Work out the finished part from the listing and answer in its coordinate system (mm). A direction names the side the tool comes from. Round coordinates to 2 decimals unless told otherwise and drop trailing zeros. Loops run counter-clockwise (first coordinate to the right, second up) from the corner with the lowest first, then second, coordinate; pieces in that order, holes last.
```python
from build123d import *

# Parameters (mm, degrees)
CUT_EXTRUDE1_START = 0.8001
CUT_EXTRUDE1_DEPTH = 14.3002
CIRPATTERN1_COUNT  = 12
SKETCH4_R          = 2.38125
CUT_EXTRUDE2_DEPTH = 34.967854094
CUT_EXTRUDE3_DEPTH = 1.7859375


with BuildPart() as part:
    # Sketch2 → Revolve1 (revolve)
    with BuildSketch(Plane(origin=(0, 0, 0), x_dir=(0, 0, -1), z_dir=(1, 0, 0)), mode=Mode.PRIVATE) as revolve1_sk:
        with BuildLine():
            Line((-15.875, 4.7625), (15.875, 4.7625))
            Line((15.875, 4.7625), (15.875, 21.2344))
            Line((15.875, 21.2344), (14.68755, 21.2344))
            ThreePointArc((14.68755, 21.2344), (13.822288491, 20.478159839), (13.5001, 19.375086298))
            Line((13.5001, 19.375086298), (13.5001, 17.515772596))
            Line((13.5001, 17.515772596), (-0.8001, 17.515772596))
            Line((-0.8001, 17.515772596), (-0.8001, 19.375086298))
            ThreePointArc((-0.8001, 19.375086298), (-1.122288491, 20.478159839), (-1.98755, 21.2344))
            Line((-1.98755, 21.2344), (-3.175, 21.2344))
            Line((-3.175, 21.2344), (-3.175, 13.5001))
            Line((-3.175, 13.5001), (-15.875, 13.5001))
            Line((-15.875, 13.5001), (-15.875, 4.7625))
        make_face()
    revolve(revolve1_sk.sketch.rotate(Axis((0, 0, 15.875), (0, 0, -1)), 90), axis=Axis((0, 0, 15.875), (0, 0, -1)))

    # Sketch3 → Cut-Extrude1 (cut)
    with BuildSketch(Plane.XY.offset(CUT_EXTRUDE1_START)):
        with BuildLine():
            Line((-1.630736704, 15.4559), (1.630736704, 15.4559))
            Line((1.630736704, 15.4559), (2.3241, 17.3609))
            ThreePointArc((2.3241, 17.3609), (0, 17.515772596), (-2.3241, 17.3609))
            Line((-2.3241, 17.3609), (-1.630736704, 15.4559))
        make_face()
    cut_extrude1 = extrude(amount=-CUT_EXTRUDE1_DEPTH, mode=Mode.SUBTRACT)

    # CirPattern1: Cut-Extrude1 ×12 about axis
    cirpattern1_axis = Axis((0, 0, 0), (0, 0, 1))
    for i in range(1, CIRPATTERN1_COUNT):
        add(cut_extrude1.rotate(cirpattern1_axis, i * 360 / CIRPATTERN1_COUNT), mode=Mode.SUBTRACT)

    # Sketch4 → Cut-Extrude2 (cut, through all)
    with BuildSketch(Plane(origin=(0, 0, 0), x_dir=(0, -1, 0), z_dir=(1, 0, 0))):
        with Locations(Location((0, -9.525, 0), (0, 0, 270))):
            Circle(SKETCH4_R)
    extrude(amount=CUT_EXTRUDE2_DEPTH, mode=Mode.SUBTRACT)

    # Sketch5 → Revolve2 (revolve)
    with BuildSketch(Plane.XY.offset(9.525)):
        Polygon((4.7625, -2.00025), (4.7625, 0), (13.288429119, 0), (13.288429119, -2.00025), (12.907429119, -2.38125), (5.1435, -2.38125), align=None)
    revolve(axis=Axis((4.7625, 0, 9.525), (1, 0, 0)))

    # Sketch6 → Cut-Extrude3 (cut)
    with BuildSketch(Plane(origin=(13.288429119, 5.384140679, 0), x_dir=(0, -1, 0), z_dir=(-1, 0, 0))):
        Polygon((5.384140679, 10.899815329), (4.193515679, 10.212407664), (4.193515679, 8.837592336), (5.384140679, 8.150184671), (6.574765679, 8.837592336), (6.574765679, 10.212407664), align=None)
    extrude(amount=CUT_EXTRUDE3_DEPTH, mode=Mode.SUBTRACT)


solid = part.part
```
1. Which of the six approach directions +Z, -Z, +X, -X, +Y, -Y give full straight-line access (tool end or side, diameter ignored) to faces 4 (the face through (-2.93, 13.18, 9.61)), 5 (the face through (-12.36, -12.41, -6.25)), 6 (the face through (15.213, -6.494, -6.25)), 7 (the face through (16.927, -4.503, -6.25))?
Answer key:
face 4: +Z
face 5: -X, -Y
face 6: -Y
face 7: +X, -Y
2. Find section A-A (x = 0). Write down the section's boundary in (y, z) (1 decimal).
Answer key:
outline: (-21.2, -15.9) - (-4.8, -15.9) - (-4.8, 15.9) - (-13.5, 15.9) - (-13.5, 3.2) - (-21.2, 3.2) - (-21.2, 2) arc R2 ccw to (-19.4, 0.8) - (-15.5, 0.8) - (-15.5, -13.5) - (-19.4, -13.5) arc R2 ccw to (-21.2, -14.7) - close; (4.8, -15.9) - (21.2, -15.9) - (21.2, -14.7) arc R2 ccw to (19.4, -13.5) - (15.5, -13.5) - (15.5, 0.8) - (19.4, 0.8) arc R2 ccw to (21.2, 2) - (21.2, 3.2) - (13.5, 3.2) - (13.5, 15.9) - (4.8, 15.9) - close
3. Given pin 1 (11 mm diameter, centred on x = 0, y = 0, fed in from +Z) (3 decimals); pin 2 (2 mm diameter, centred on x = 8, z = 11.5, fed in from +Y); pin 3 (12 mm diameter, centred on y = 2, z = -4.5, fed in from +X); pin 4 (1.5 mm diameter, centred on x = 12.5, z = 10, fed in from -Y), each flat-ended and moving along its own axis, determine where each tip first touches the part or whether it passes through.
Answer key:
pin 1: stops at z = 15.875
pin 2: stops at y = 11.54
pin 3: stops at x = 20.85
pin 4: stops at y = -6.65
4. Consider probe 1 along X at (y, z) = (13, -7); probe 2 along Z at (x, y) = (-12.5, -14.5) (3 decimals); probe 3 along Z at (x, y) = (4, -16) (3 decimals). Determine where each line is inside the solid, lowest interval first.
Answer key:
probe 1: x = -11.74 to -9.65, -8.4 to 8.4, 9.65 to 11.74
probe 2: z = -15.875 to -13.5, 0.8 to 3.175
probe 3: z = -15.875 to 3.175
5. Determine the mould class of faces 1 (the face through (1.973, 16.395, -6.25)), 2 (the face through (-2.764, -21.054, -15.273)), 3 (the face through (12.408, -0.604, 10.551)) for opening direction Y: +Y half, -Y half, draft (parallel to the pull), parting line (faces both ways), or undercut.
Answer key:
face 1: +Y half
face 2: parting line
face 3: undercut
